```python
from build123d import *

# Parameters (mm, degrees)
SKETCH1_R           = 5
BOSS_EXTRUDE1_DEPTH = 85
SKETCH2_R           = 2
CUT_EXTRUDE1_DEPTH  = 15
CUT_EXTRUDE2_DEPTH  = 10
SKETCH4_R           = 2
CUT_EXTRUDE3_DEPTH  = 6.165903358


with BuildPart() as part:
    # Sketch1 → Boss-Extrude1 (new body)
    with BuildSketch(Plane(origin=(0, 0, 0), x_dir=(1, 0, 0), z_dir=(0, 1, 0))):
        Circle(SKETCH1_R)
    extrude(amount=BOSS_EXTRUDE1_DEPTH)

    # Sketch2 → Cut-Extrude1 (cut)
    with BuildSketch(Plane(origin=(0, 85, 0), x_dir=(1, 0, 0), z_dir=(0, 1, 0))):
        Circle(SKETCH2_R)
    extrude(amount=-CUT_EXTRUDE1_DEPTH, mode=Mode.SUBTRACT)

    # Sketch3 → Cut-Extrude2 (cut)
    with BuildSketch(Plane.XZ):
        with BuildLine():
            Line((-5, 0), (4.997224535, 0.166574151))
            ThreePointArc((4.997224535, 0.166574151), (-0.084674808, 5.081899343), (-5, 0))
        make_face()
    extrude(amount=-CUT_EXTRUDE2_DEPTH, mode=Mode.SUBTRACT)

    # Sketch4 → Cut-Extrude3 (cut, through all)
    with BuildSketch(Plane(origin=(-0.001387733, 0, 0.083287076), x_dir=(0.999861217, 0, 0.016659727), z_dir=(-0.016659727, 0, 0.999861217))):
        with Locations((0, 5)):
            Circle(SKETCH4_R)
    extrude(amount=-CUT_EXTRUDE3_DEPTH, mode=Mode.SUBTRACT)


solid = part.part
```
The model under review builds one solid part; all positions refer to its coordinate system, in mm. A direction names the side the tool comes from. Give positions to 0.01 mm unless a question says otherwise; leave off trailing zeros. Write each loop counter-clockwise with the first axis right and the second up, starting at its lowest first coordinate (ties: lowest second). Pieces come first, ordered by that corner, then holes. Notation, with made-up numbers: (-23.75, -1.75) -> (-9.75, -1.75) arc R21 ccw to (-9.75, 7.25) -> close; hole circle Ø3 at (69, 66). An arc over 180 degrees is marked (long way). Answer in a Markdown table with one row per item.
1) Add section D-D on x = -3.25. State the section outline as (y, z) points, plus the area to 3 significant figures.
Worked answers:
| item | result |
|---|---|
| outline | (0, -3.8) -> (85, -3.8) -> (85, 3.8) -> (10, 3.8) -> (10, 0.03) -> (0, 0.03) -> close |
| area | 608 mm² |
2) Add section C-C on z = 1.25. State the section outline as (x, y) points, plus the area to 3 significant figures.
Worked answers:
| item | result |
|---|---|
| outline | (-4.84, 10) -> (4.84, 10) -> (4.84, 85) -> (1.56, 85) -> (1.56, 70) -> (-1.56, 70) -> (-1.56, 85) -> (-4.84, 85) -> close |
| area | 679 mm² |
3) Tool access review of faces 1 (the flat face through (0, 70, 0)), 2 (the flat face through (0, 0, -2)): name each direction out of +Z, -Z, +X, -X, +Y, -Y from which nothing blocks a thin tool from reaching the whole face with its end or side.
Worked answers:
| item | result |
|---|---|
| face 1 | +Y |
| face 2 | +Z, -Z, +X, -X, -Y |
4) For L1, parallel to X at y = 74.25, z = 0; L2, parallel to Y at x = 1.5, z = 2.25, list the stretches that pass through material, from the lowest coordinate up. Write a range as [from, to].
Worked answers:
| item | result |
|---|---|
| L1 | [-5, -2], [2, 5] |
| L2 | [10, 85] |
5) Clearance check with flat-ended pins moving along their axes: P1, Ø5, axis at y = 21, z = 4, coming from the +X side; P2, Ø4, axis at x = -3, y = 59, coming from the +Z side. State where each tip first meets the part, or that it passes through.
Worked answers:
| item | result |
|---|---|
| P1 | x = 4.77 |
| P2 | z = 4.9 |
6) Add section B-B on y = 20. State the section outline as (x, z) points.
Worked answers:
| item | result |
|---|---|
| outline | circle Ø10 at (0, 0) |
7) Add section A-A on y = 76.5. State the section outline as (x, z) points, plus the area to 3 significant figures.
Worked answers:
| item | result |
|---|---|
| outline | circle Ø10 at (0, 0); hole circle Ø4 at (0, 0) |
| area | 66.0 mm² |
8) Mouldability with a two-part tool opening along X and no side actions: class faces 3 (the flat face through (0, 10, 2)), 4 (the cylindrical face through (0, 78, 2)), 5 (the cylindrical face through (-0.651, 41.905, -4.957)), 6 (the cylindrical face through (-1.957, 5.088, -2.457)) as +X half, -X half, draft (parallel to the pull), parting line (faces both ways), or undercut.
Worked answers:
| item | result |
|---|---|
| face 3 | draft |
| face 4 | undercut |
| face 5 | parting line |
| face 6 | undercut |
